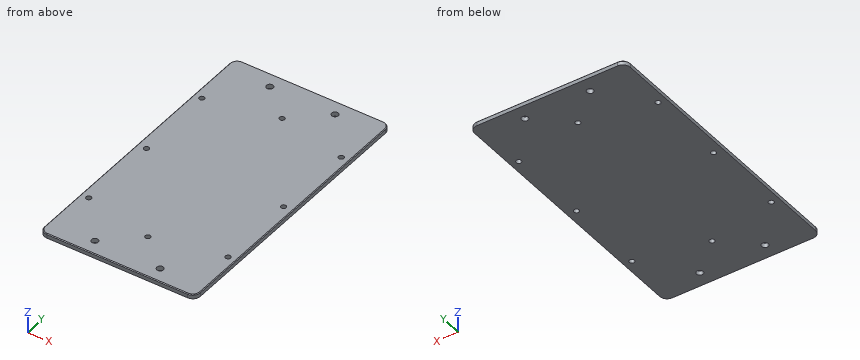
Autodesk Inventor part; units mm, degrees
ref_plane "YZ Plane" through (0, 0, 0) normal (1, 0, 0) x (0, 1, 0)
ref_plane "XZ Plane" through (0, 0, 0) normal (0, 1, 0) x (-1, 0, 0)
ref_plane "XY Plane" through (0, 0, 0) normal (0, 0, 1) x (1, 0, 0)
sketch "Sketch1" plane through (0, 0, 0) normal (0, 0, 1) x (1, 0, 0)
  line L0 (-52.5, -95) -> (52.5, -95)
  line L1 (52.5, -95) -> (52.5, 95)
  line L2 (52.5, 95) -> (-52.5, 95)
  line L3 (-52.5, 95) -> (-52.5, -95)
  line L4 (-52.5, -95) -> (52.5, 95) construction
  line L5 (52.5, -95) -> (-52.5, 95) construction
  point P0 (0, 0)
  dimension "d0" = 190
  dimension "d1" = 105
extrude "Extrusion1" add sketch "Sketch1" along normal blind 3
sketch "Sketch2" plane through (0, 0, 3) normal (0, 0, 1) x (1, 0, 0)
  circle A0 centre (-47, 55) radius 1.75
  line L0 (-52.5, 95) -> (-52.5, -95) construction
  line L1 (-73.5, 0) -> (73.5, 0)
  line L2 (0, 133) -> (0, -133)
  circle A1 centre (47, 55) radius 1.75
  circle A2 centre (-47, -55) radius 1.75
  circle A3 centre (47, -55) radius 1.75
  point P0 (0, 0)
  point P1 (52.5, 95)
  point P2 (52.5, -95)
  dimension "d6" = 47
  dimension "d7" = 3.5
  dimension "d8" = 55
extrude "Extrusion2" cut sketch "Sketch2" against normal blind 3
sketch "Sketch3" plane through (0, 0, 3) normal (0, 0, 1) x (1, 0, 0)
  circle A0 centre (-22, 85) radius 2.25
  line L0 (52.5, 95) -> (-52.5, 95) construction
  line L1 (0, 133) -> (0, -133)
  line L2 (-73.5, 0) -> (73.5, 0)
  circle A1 centre (22, 85) radius 2.25
  circle A2 centre (-22, -85) radius 2.25
  line L3 (52.5, -95) -> (-52.5, -95) construction
  circle A3 centre (22, -85) radius 2.25
  point P0 (0, 0)
  dimension "d11" = 10
  dimension "d12" = 4.5
extrude "Extrusion3" cut sketch "Sketch3" against normal blind 3
sketch "Sketch4" plane through (0, 0, 3) normal (0, 0, 1) x (1, 0, 0)
  line L0 (-40, -59) -> (40, -59) construction
  line L1 (40, -59) -> (40, 59) construction
  line L2 (40, 59) -> (-40, 59) construction
  line L3 (-40, 59) -> (-40, -59) construction
  line L4 (-40, -59) -> (40, 59) construction
  line L5 (40, -59) -> (-40, 59) construction
  line L6 (-73.5, 0) -> (73.5, 0) construction
  line L7 (0, -133) -> (0, 133) construction
  circle A0 centre (0, 65.25) radius 1.75
  circle A1 centre (-46.25, 0) radius 1.75
  circle A2 centre (0, -65.25) radius 1.75
  circle A3 centre (46.25, 0) radius 1.75
  line L8 (-52.5, 95) -> (-52.5, -95)
  circle A4 centre (-47, -55) radius 1.75
  circle A5 centre (-47, 55) radius 1.75
  point P0 (0, 0)
  dimension "d15" = 80
  dimension "d16" = 118
  dimension "d17" = 3.5
  dimension "d18" = 3.5
  dimension "d19" = 12.5
  dimension "d21" = 6.25
  dimension "d24" = 6.25
  dimension "d29" = 110
extrude "Extrusion4" cut sketch "Sketch4" against normal blind 3 contours A0 | A1 | A2 | A3
fillet "Fillet1" radius 5 4 edges at (-52.5, -95, 1.5) (52.5, -95, 1.5) (52.5, 95, 1.5) (-52.5, 95, 1.5)
chamfer "Chamfer1" distance 0.5 angle 45 8 edges at (-52.5, 0, 3) (-51.0355, -93.5355, 3) (0, -95, 3) (51.0355, -93.5355, 3) (52.5, 0, 3) (51.0355, 93.5355, 3) (0, 95, 3) (-51.0355, 93.5355, 3)
equation "\"d18\" = d17"
equation "\"d21\" = d24"
equation "\"d24\" = 0.5 * d19"
properties part number "BatteryHolderBottom"
The model under review builds one solid part; all positions refer to its coordinate system, in mm. Give positions to 0.01 mm unless a question says otherwise; leave off trailing zeros. Write each loop counter-clockwise with the first axis right and the second up, starting at its lowest first coordinate (ties: lowest second). Pieces come first, ordered by that corner, then holes. Notation, with made-up numbers: (-8, 19) -> (38, 19) arc R29 cw to (38, 47) -> close; hole circle Ø10 at (12, 71.25). An arc over 180 degrees is marked (long way). Answer in a Markdown table with one row per item.
1) Clearance check with a flat-ended pin moving along its axis: P1, Ø4, axis at x = 22, y = 85, coming from the +Z side. State where the tip first meets the part, or that it passes through.
Worked answers:
| item | result |
|---|---|
| P1 | through |
2) Add section C-C on y = 65.25. State the section outline as (x, z) points, plus the area to 3 significant figures.
Worked answers:
| item | result |
|---|---|
| outline | (-52.5, 0) -> (-1.75, 0) -> (-1.75, 3) -> (-52, 3) -> (-52.5, 2.5) -> close; (1.75, 0) -> (52.5, 0) -> (52.5, 2.5) -> (52, 3) -> (1.75, 3) -> close |
| area | 304 mm² |
3) For L1, parallel to Y at x = -22, z = 0.9; L2, parallel to Y at x = 0, z = 1.7; L3, parallel to Y at x = 47, z = 1.05, list the stretches that pass through material, from the lowest coordinate up. Write a range as [from, to].
Worked answers:
| item | result |
|---|---|
| L1 | [-95, -87.25], [-82.75, 82.75], [87.25, 95] |
| L2 | [-95, -67], [-63.5, 63.5], [67, 95] |
| L3 | [-95, -56.75], [-53.25, -1.58], [1.58, 53.25], [56.75, 95] |
4) Add section B-B on y = 0. State the section outline as (x, z) points.
Worked answers:
| item | result |
|---|---|
| outline | (-52.5, 0) -> (-48, 0) -> (-48, 3) -> (-52, 3) -> (-52.5, 2.5) -> close; (-44.5, 0) -> (44.5, 0) -> (44.5, 3) -> (-44.5, 3) -> close; (48, 0) -> (52.5, 0) -> (52.5, 2.5) -> (52, 3) -> (48, 3) -> close |
5) Add section A-A on x = 22. State the section outline as (y, z) points.
Worked answers:
| item | result |
|---|---|
| outline | (-95, 0) -> (-87.25, 0) -> (-87.25, 3) -> (-94.5, 3) -> (-95, 2.5) -> close; (-82.75, 0) -> (82.75, 0) -> (82.75, 3) -> (-82.75, 3) -> close; (87.25, 0) -> (95, 0) -> (95, 2.5) -> (94.5, 3) -> (87.25, 3) -> close |
